Drawing for the job (mm, zero at the part's lowest x, y, z). Give positions to 0.01 mm unless a question says otherwise; leave off trailing zeros. Order: outer loops, then holes, each group sorted by start corner. A loop starts at its lowest first (then second) coordinate and runs counter-clockwise, first axis right, second up. Notation, with made-up numbers: (49.5, -29) - (108.5, -29) arc R28 cw to (108.5, -8) - close; hole circle Ø5 at (-37, 87). An arc over 180 degrees is marked (long way). One line per item, written item: value.
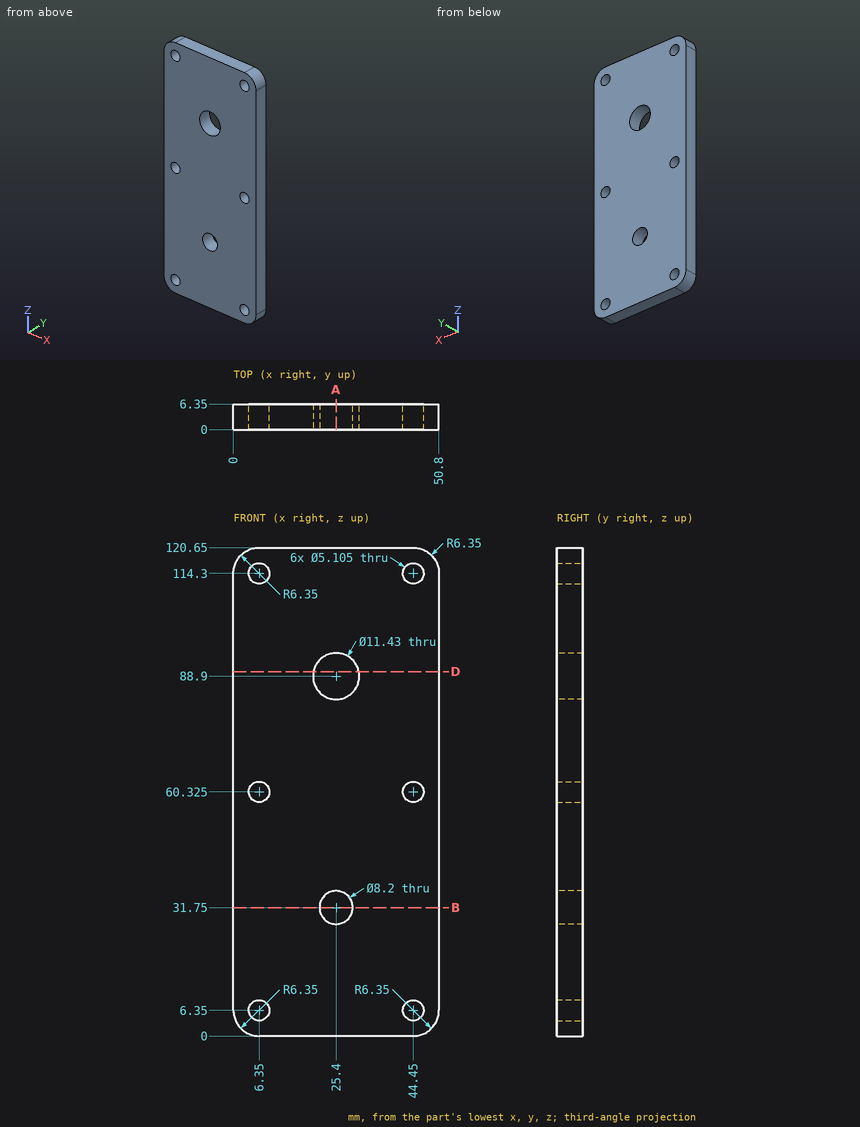
1) Pin check, flat tip, straight feed: pin 1 (3 mm diameter, centred on x = 6.35, z = 114.3, fed in from +Y). Stop position of the tip, or through.
Outcome:
pin 1: passes through
2) Drill centre lines: line 1 along Z through (x, y) = (6.35, 5.25); line 2 along Z through (x, y) = (25.5, 3); line 3 along X through (y, z) = (5, 112.5). Where is each one in solid material? Low to high. Write a range as from..to.
Outcome:
line 1: z = 0..3.8, 8.9..57.77, 62.88..111.75, 116.85..120.65
line 2: z = 0..27.65, 35.85..83.19, 94.61..120.65
line 3: x = 0..4.54, 8.16..42.64, 46.26..50.8
3) Cut at D-D, the plane z = 90. Give the cut face in (x, y), then the cut area to 3 significant figures.
Outcome:
outline: (0, 0) - (19.79, 0) - (19.79, 6.35) - (0, 6.35) - close; (31.01, 0) - (50.8, 0) - (50.8, 6.35) - (31.01, 6.35) - close
area: 251 mm^2
4) Cut at A-A, the plane x = 25.4. Give the number of separate pieces and of enclosed holes in the cut face.
Outcome:
separate pieces: 3
enclosed holes: 0
5) Cut at B-B, the plane z = 31.75. Give the cut face in (x, y).
Outcome:
outline: (0, 0) - (21.3, 0) - (21.3, 6.35) - (0, 6.35) - close; (29.5, 0) - (50.8, 0) - (50.8, 6.35) - (29.5, 6.35) - close
